Input: part model. Units: mm. Frame: model coordinates. Coordinates: 2 decimals unless noted, no trailing zeros. Write each loop counter-clockwise with the first axis right and the second up, starting at its lowest first coordinate (ties: lowest second). Pieces come first, ordered by that corner, then holes.
1) Line query: L1, parallel to Z at x = 0, y = 38; L2, parallel to Z at x = 0, y = 18; L3, parallel to Y at x = -6.5, z = -33. Output: solid intervals per line, ascending.
2) Section query A-A (x = 0). Output: boundary loops of the cut face in (y, z).
3) Draft query along Z for faces 1 (the flat face through (-5, 50.8, 12)), 2 (the cylindrical face through (-0.559, 12.522, -101.594)), 3 (the cylindrical face through (-11.721, 30.689, 22.534)), 4 (the cylindrical face through (2.75, 25.04, 12.4)). Return one class per face: pulls with the +Z half, pulls with the -Z half, needs draft (parallel to the pull), parting line crosses it, or undercut.
4) Section query B-B (z = -8). Output: boundary loops of the cut face in (x, y).
5) Section query D-D (x = 17). Output: boundary loops of the cut face in (y, z), then the cut area to 3 significant figures.
6) Section query C-C (y = 30.5). Output: boundary loops of the cut face in (x, z).
7) Pin query (flat end, axial travel): pin 1 Ø1.5 at (x, y) = (2.5, 10.5) entering from +Z; pin 2 Ø6 at (x, y) = (-14.5, 34) entering from -Z; pin 3 Ø6 at (y, z) = (9, -82.5) entering from -X. Return the tip coordinate at first contact, or that it passes through.
Autodesk Inventor part; units mm, degrees
ref_plane "YZ Plane" through (0, 0, 0) normal (1, 0, 0) x (0, 1, 0)
ref_plane "XZ Plane" through (0, 0, 0) normal (0, 1, 0) x (-1, 0, 0)
ref_plane "XY Plane" through (0, 0, 0) normal (0, 0, 1) x (1, 0, 0)
sketch "Sketch1" plane through (0, 0, 0) normal (0, 1, 0) x (-1, 0, 0)
  circle A0 centre (0, 0) radius 25.4
  line L0 (-25.4, 0) -> (-25.4, -76.2)
  line L1 (25.4, -76.2) -> (25.4, 0)
  arc A1 (-25.4, -76.2) -> (25.4, -76.2) centre (0, -76.2) ccw
  circle A2 centre (0, 0) radius 12.7
  dimension "d0" = 50.8
  dimension "d1" = 76.2
  dimension "d2" = 50.8
  dimension "d3" = 25.4
extrude "Extrusion1" add sketch "Sketch1" along normal blind 25.4 contours L1 A1 L0 A0
extrude "Extrusion2" add sketch "Sketch1" along normal blind 50.8 contours A0
properties part number "10-18-19 D"
Answer:
1. L1: z = -25.4 to -12.7, 12.7 to 25.4
1. L2: z = -101.6 to -12.7, 12.7 to 25.4
1. L3: y = 0 to 25.4
2. outline: (0, -101.6) - (25.4, -101.6) - (25.4, -25.4) - (50.8, -25.4) - (50.8, -12.7) - (0, -12.7) - close; (0, 12.7) - (50.8, 12.7) - (50.8, 25.4) - (0, 25.4) - close
3. face 1: needs draft
3. face 2: pulls with the -Z half
3. face 3: parting line crosses it
3. face 4: undercut
4. outline: (-25.4, 0) - (-9.86, 0) - (-9.86, 50.8) - (-24.11, 50.8) - (-24.11, 25.4) - (-25.4, 25.4) - close; (9.86, 0) - (25.4, 0) - (25.4, 25.4) - (24.11, 25.4) - (24.11, 50.8) - (9.86, 50.8) - close
5. outline: (0, -95.07) - (25.4, -95.07) - (25.4, -18.87) - (50.8, -18.87) - (50.8, 18.87) - (0, 18.87) - close
5. area: 3,850 mm2
6. outline: circle Ø50.8 at (0, 0); hole circle Ø25.4 at (0, 0)
7. pin 1: stops at z = 25.34
7. pin 2: stops at z = -22.65
7. pin 3: stops at x = -25.18
